Geometry check sheet. Reference: the model listing, model coordinates, mm. A direction names the side the tool comes from. Coordinates: 2 decimals unless noted, no trailing zeros. Write each loop counter-clockwise with the first axis right and the second up, starting at its lowest first coordinate (ties: lowest second). Pieces come first, ordered by that corner, then holes. Notation, with made-up numbers: (-25.5, 33.5) -> (-6.5, 33.5) arc R25 cw to (-6.5, 61.5) -> close; hole circle Ø7 at (62, -23.75). An arc over 180 degrees is marked (long way). One line per question, with ' | ' between items.
Autodesk Inventor part; units mm, degrees
ref_plane "YZ Plane" through (0, 0, 0) normal (1, 0, 0) x (0, 1, 0)
ref_plane "XZ Plane" through (0, 0, 0) normal (0, 1, 0) x (-1, 0, 0)
ref_plane "XY Plane" through (0, 0, 0) normal (0, 0, 1) x (1, 0, 0)
sketch "スケッチ1" plane through (0, 0, 0) normal (1, 0, 0) x (0, 1, 0)
  line L0 (0, 13) -> (0, 0)
  line L1 (0, 0) -> (2.25, 0)
  line L2 (2.25, 0) -> (2.25, 3)
  line L3 (2.25, 3) -> (1.5, 3)
  line L4 (1.5, 3) -> (1.5, 13)
  line L5 (1.5, 13) -> (0, 13)
  dimension "d2" = 3
  dimension "d10" = 10
  dimension "d11" = 3
  dimension "d12" = 4.5
revolve "回転1" add sketch "スケッチ1" angle 360 about axis through (0, 0, 13) along (0, 0, -1)
thread "ねじ1"
sketch "スケッチ2" plane through (0, 0, 0) normal (0, 0, -1) x (-1, 0, 0)
  line L0 (0, 1.4434) -> (1.25, 0.7217)
  line L1 (1.25, 0.7217) -> (1.25, -0.7217)
  line L2 (1.25, -0.7217) -> (0, -1.4434)
  line L3 (0, -1.4434) -> (-1.25, -0.7217)
  line L4 (-1.25, -0.7217) -> (-1.25, 0.7217)
  line L5 (-1.25, 0.7217) -> (0, 1.4434)
  circle A0 centre (0, 0) radius 2.25
  line L6 (0, 2.25) -> (0, -2.25) construction
  point P0 (0, 0)
  dimension "d7" = 2.5
extrude "押し出し1" cut sketch "スケッチ2" against normal blind 1.4 contours L0 L1 L2 L3 L4 L5
properties part number "CSHSM-SUS-M3-10" material "ステンレス鋼 AISI 304"
(1) Draft check along Y on faces 4 (the face through (-0.07, -1.5, 8.07)), 5 (the face through (-1.25, 0, 1)), 6 (the face through (-1.5, 0, 0)). Enter one of: pulls with the +Y half, pulls with the -Y half, needs draft (parallel to the pull), parting line crosses it, or undercut.
Answers below:
face 4: parting line crosses it | face 5: undercut | face 6: needs draft
(2) Cross-section at B-B (y = 0). Record the cut outline in (x, z), plus the area to 3 significant figures.
Answers below:
outline: (-2.25, 0) -> (-1.25, 0) -> (-1.25, 1.4) -> (1.25, 1.4) -> (1.25, 0) -> (2.25, 0) -> (2.25, 3) -> (1.5, 3) -> (1.5, 13) -> (-1.5, 13) -> (-1.5, 3) -> (-2.25, 3) -> close | area: 40.0 mm²
(3) Cross-section at D-D (z = 10). Record the cut outline in (x, y), plus the area to 3 significant figures.
Answers below:
outline: circle Ø3 at (0, 0) | area: 7.07 mm²
(4) Tool access check on faces 1 (the face through (0, -2, 3)), 2 (the face through (-2.23, -0.29, 1.52)), 3 (the face through (0, 0, 1.4)). Record the directions out of +Z, -Z, +X, -X, +Y, -Y that give a thin tool (end or side, any length) a straight path to the whole face; none if there is none.
Answers below:
face 1: +Z | face 2: +Z, -Z | face 3: -Z
(5) Material ranges on line 1 (Z direction, x = -1.8, y = 1.05); line 2 (Z direction, x = -0.85, y = -0.6); line 3 (Y direction, x = -0.05, z = 4), recorded low to high.
Answers below:
line 1: z = 0 to 3 | line 2: z = 1.4 to 13 | line 3: y = -1.5 to 1.5
(6) Cross-section at C-C (z = 1.75). Record the cut outline in (x, y), plus the area to 3 significant figures.
Answers below:
outline: circle Ø4.5 at (0, 0) | area: 15.9 mm²
(7) Cross-section at A-A (x = 0.8). Record the cut outline in (y, z).
Answers below:
outline: (-2.1, 0) -> (-0.98, 0) -> (-0.98, 1.4) -> (0.98, 1.4) -> (0.98, 0) -> (2.1, 0) -> (2.1, 3) -> (1.27, 3) -> (1.27, 13) -> (-1.27, 13) -> (-1.27, 3) -> (-2.1, 3) -> close
(8) Depth check by flat-ended pin: P1, Ø1.5, axis at y = -1.5, z = 7, coming from the -X side; P2, Ø2, axis at y = 0.5, z = 11, coming from the +X side. Enter the tip coordinate at first touch or a pass-through.
Answers below:
P1: stops at x = -1.3 | P2: stops at x = 1.5
